Part print with two shaded views. Sizes in mm from the minimum x, y, z corner. Coordinates: 2 decimals unless noted, no trailing zeros. Write each loop counter-clockwise with the first axis right and the second up, starting at its lowest first coordinate (ties: lowest second). Pieces come first, ordered by that corner, then holes. Notation, with made-up numbers: (69, 27) - (93, 27) arc R13 ccw to (93, 41) - close; hole circle Ø3 at (1, 33.25). An arc over 180 degrees is marked (long way). Answer in a Markdown table with one row per item. Add a question column.
Q1. Band-saw the part on C-C (y = 3). List the corners of the cut face in (x, z) (3 decimals), and give its area (3 significant figures).
Q2. Band-saw the part on B-B (y = 50.5). List the corners of the cut face in (x, z), and give its area (3 significant figures).
Q3. Band-saw the part on D-D (x = 27). List the corners of the cut face in (y, z) (3 decimals), and give its area (3 significant figures).
Q4. Pin check, flat tips, straight feed: pin 1 (5.5 mm diameter, centred on x = 27, y = 3, fed in from +Z); pin 2 (3 mm diameter, centred on y = 95, z = 4.5, fed in from +X); pin 3 (1 mm diameter, centred on x = 39.5, y = 98.5, fed in from -Z). Stop position of each tip, or through.
Q5. Drill centre lines: line 1 along X through (y, z) = (63, 4.3); line 2 along Y through (x, z) = (18, 1); line 3 along X through (y, z) = (38, 3.1). Where is each one in solid material? Low to high. Write a range as from..to.
Q6. Band-saw the part on A-A (x = 40). List the corners of the cut face in (y, z).
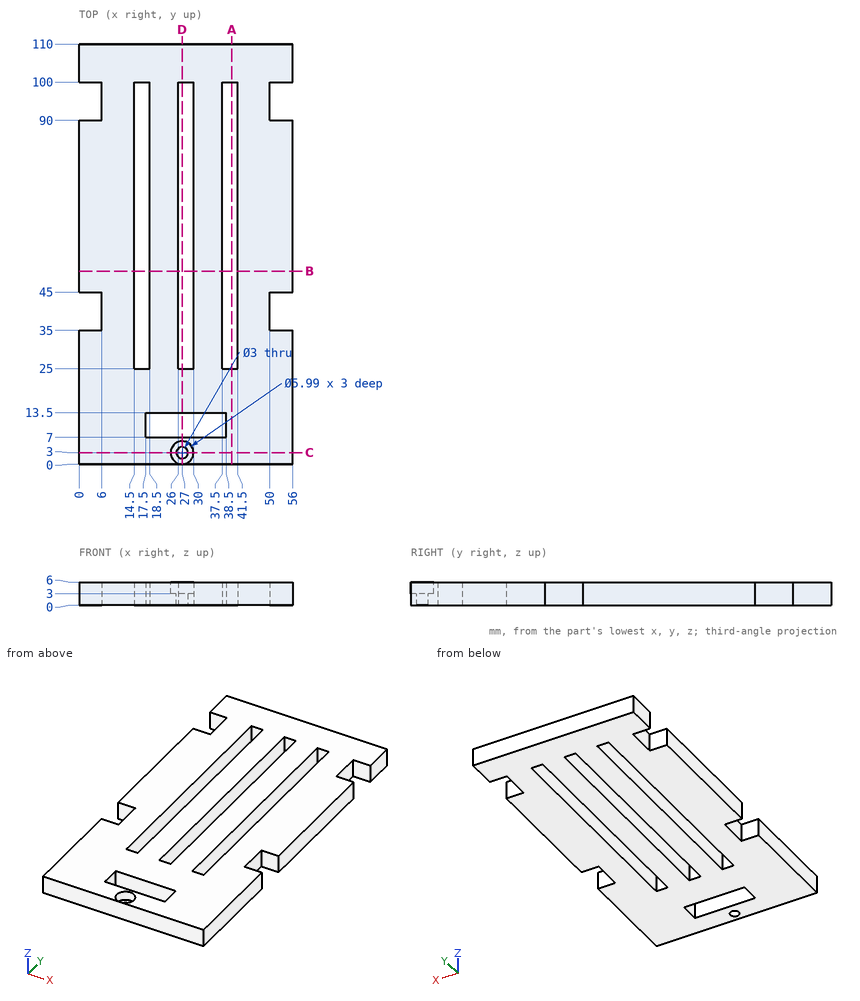
Checked values:
| question | item | result |
|---|---|---|
| 1 | outline | (0, 0) - (25.5, 0) - (25.5, 3) - (24.005, 3) - (24.005, 6) - (0, 6) - close; (28.5, 0) - (56, 0) - (56, 6) - (29.995, 6) - (29.995, 3) - (28.5, 3) - close |
| 1 | area | 309 mm² |
| 2 | outline | (0, 0) - (14.5, 0) - (14.5, 6) - (0, 6) - close; (18.5, 0) - (26, 0) - (26, 6) - (18.5, 6) - close; (30, 0) - (37.5, 0) - (37.5, 6) - (30, 6) - close; (41.5, 0) - (56, 0) - (56, 6) - (41.5, 6) - close |
| 2 | area | 264 mm² |
| 3 | outline | (0, 0) - (1.5, 0) - (1.5, 3) - (0.005, 3) - (0.005, 6) - (0, 6) - close; (4.5, 0) - (7, 0) - (7, 6) - (5.995, 6) - (5.995, 3) - (4.5, 3) - close; (13.5, 0) - (25, 0) - (25, 6) - (13.5, 6) - close; (100, 0) - (110, 0) - (110, 6) - (100, 6) - close |
| 3 | area | 144 mm² |
| 4 | pin 1 | stops at z = 3 |
| 4 | pin 2 | stops at x = 50 |
| 4 | pin 3 | passes through |
| 5 | line 1 | x = 0..14.5, 18.5..26, 30..37.5, 41.5..56 |
| 5 | line 2 | y = 0..7, 13.5..25, 100..110 |
| 5 | line 3 | x = 6..14.5, 18.5..26, 30..37.5, 41.5..50 |
| 6 | outline | (0, 0) - (25, 0) - (25, 6) - (0, 6) - close; (100, 0) - (110, 0) - (110, 6) - (100, 6) - close |
